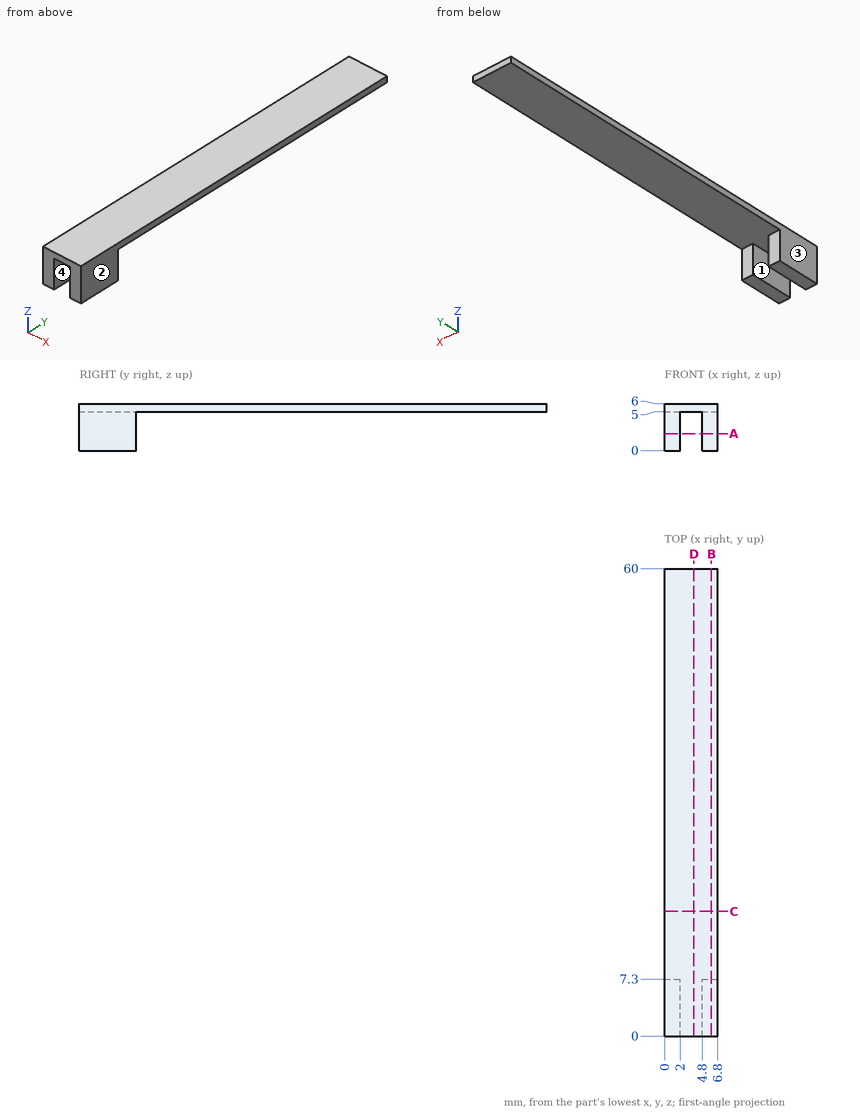
For this review, use the dimensioned drawing (mm, ordinates from the lowest corner) and the shaded views. Round coordinates to 2 decimals unless told otherwise and drop trailing zeros. Write each loop counter-clockwise with the first axis right and the second up, starting at its lowest first coordinate (ties: lowest second). Pieces come first, ordered by that corner, then holes. Notation, with made-up numbers: M -5,-38.5 L 50,-38.5 A26 ccw 50,-10.5 Z; hole C -38,12.5 d8. An arc over 180 degrees is marked long. Write item = value, one per line. Start each with the question number.
(1) Clearance check with flat-ended pins moving along their axes: pin 1 Ø3 at (x, y) = (5, 46.5) entering from -Z; pin 2 Ø1.6 at (x, z) = (0.5, 2) entering from +Y; pin 3 Ø1.5 at (y, z) = (29, 3.5) entering from -X. State where each tip first meets the part, or that it passes through.
(2) We need section B-B (x = 6). Give the boundary of the cut face in (y, z), then the cut area to 3 significant figures.
(3) The part is to be moulded in two halves that separate along X. For the marked faces 1, 2, 3 and 4, say which applies: +X half, -X half, draft (parallel to the pull), parting line (faces both ways), or undercut.
(4) We need section C-C (y = 16). Give the boundary of the cut face in (x, z).
(5) For line 1 along Y through (x, z) = (1.25, 2.4); line 2 along X through (y, z) = (3.5, 3.1); line 3 along Z through (x, y) = (3.75, 20), list the stretches that pass through material, from the lowest coordinate up.
(6) We need section A-A (z = 2.2). Give the boundary of the cut face in (x, y), then the cut area to 3 significant figures.
(7) We need section D-D (x = 3.75). Give the boundary of the cut face in (y, z), then the cut area to 3 significant figures.
Results found:
q1.pin_1 = 5
q1.pin_2 = 7.3
q1.pin_3 = through
q2.outline = M 0,0 L 7.3,0 L 7.3,5 L 60,5 L 60,6 L 0,6 Z
q2.area = 96.5 mm²
q3.face_1 = undercut
q3.face_2 = +X half
q3.face_3 = -X half
q3.face_4 = undercut
q4.outline = M 0,5 L 6.8,5 L 6.8,6 L 0,6 Z
q5.line_1 = 0 to 7.3
q5.line_2 = 0 to 2, 4.8 to 6.8
q5.line_3 = 5 to 6
q6.outline = M 0,0 L 2,0 L 2,7.3 L 0,7.3 Z; M 4.8,0 L 6.8,0 L 6.8,7.3 L 4.8,7.3 Z
q6.area = 29.2 mm²
q7.outline = M 0,5 L 60,5 L 60,6 L 0,6 Z
q7.area = 60.0 mm²
